Work out the finished part from the listing and answer in its coordinate system (mm). A direction names the side the tool comes from. Coordinates: 2 decimals unless noted, no trailing zeros. Order: outer loops, then holes, each group sorted by start corner. A loop starts at its lowest first (then second) coordinate and runs counter-clockwise, first axis right, second up.
1. The part is cut by section C-C, the plane z = -23.5. Give the vertices of the cut face in (x, y), then the cut area to 3 significant figures.
2. Find the intervals of material crossed by probe 1 along Y at (x, z) = (-29, -1.5); probe 2 along Z at (x, y) = (4.5, -23); probe 3 along Z at (x, y) = (6.5, -37.5), in increasing order.
3. Flat-ended cylindrical pins translate along their axes: pin 1 Ø2.5 at (y, z) = (-8, 23.5) entering from +X; pin 2 Ø3 at (x, z) = (15.34, 2.19) entering from +Y; pin 3 Ø2 at (x, y) = (-28.5, -6) entering from -Z; pin 4 Ø1.5 at (x, y) = (-9.5, -8) entering from +Z. Find the tip coordinate at first contact, or state that the pin passes through.
4. A tool of negligible diameter and unlimited length cuts with its end or side. For faces 1 (the flat face through (3.5, -38, 24)), 2 (the flat face through (16.084, 2, 14)), 3 (the flat face through (-32.5, -6, 0)), from which of +Z, -Z, +X, -X, +Y, -Y can it reach the whole face along a straight path? Write none if from no direction.
5. The part is cut by section D-D, the plane y = -4. Give the vertices of the cut face in (x, z).
6. The part is cut by section B-B, the plane y = -38. Give the vertices of the cut face in (x, z).
7. The part is cut by section A-A, the plane x = -5.5. Give the vertices of the cut face in (y, z), then the cut area to 3 significant figures.
8. Determine the mould class of faces 4 (the flat face through (-29, -20, 0)), 5 (the flat face through (-30, -6, -10)), 6 (the flat face through (9, -23, -18.5)) for opening direction Z: +Z half, -Z half, draft (parallel to the pull), parting line (faces both ways), or undercut.
Autodesk Inventor part; units mm, degrees
ref_plane "YZ Plane" through (0, 0, 0) normal (1, 0, 0) x (0, 1, 0)
ref_plane "XZ Plane" through (0, 0, 0) normal (0, 1, 0) x (-1, 0, 0)
ref_plane "XY Plane" through (0, 0, 0) normal (0, 0, 1) x (1, 0, 0)
sketch "Sketch1" plane through (0, 0, 0) normal (0, 1, 0) x (-1, 0, 0)
  circle A0 centre (0, 0) radius 18.5
  line L0 (5.5131, -10.5135) -> (5.5131, 1.8865)
  circle A1 centre (5.5131, -4.3135) radius 6.2
  line L1 (0, 0) -> (-24.4, 0)
  circle A2 centre (5.5131, -4.3135) radius 3
  circle A3 centre (5.5131, -4.3135) radius 40
  line L2 (-24.4, 0) -> (-24.4, -81.1676)
  line L3 (-24.4, -81.1676) -> (-24.4, 62.3764)
  line L4 (0, 0) -> (0, 28.5)
  line L5 (18.5, 0) -> (28.5, 0)
  line L6 (0, -18.5) -> (0, -28.5)
  arc A4 (28.5, 0) -> (0, 28.5) centre (0, 0) ccw
  arc A5 (0, -28.5) -> (28.5, 0) centre (0, 0) ccw
  line L7 (0, 18.5) -> (0, 23.5)
  line L8 (0, 18.5) -> (-18.5, 18.5)
  line L9 (-18.5, 18.5) -> (-18.5, 28.5)
  line L10 (-18.5, 28.5) -> (0, 28.5)
  line L11 (0, -18.5) -> (-18.5, -18.5)
  line L12 (-18.5, -18.5) -> (-18.5, -28.5)
  line L13 (-18.5, -28.5) -> (0, -28.5)
  line L14 (5.5131, -4.3135) -> (-72.1542, -4.3135)
  line L15 (0, 0) -> (5.5051, -4.3135)
  line L16 (0, 0) -> (6.9938, 0) construction
  line L17 (-16.0843, 18.5) -> (-16.0843, -18.5)
  circle A6 centre (0, 0) radius 15.5
  circle A7 centre (5.5051, -4.3135) radius 24.193
  circle A8 centre (5.5051, -4.3135) radius 10.066
  circle A9 centre (15.3445, -2.1897) radius 1.75
  circle A10 centre (9.5686, 12.1939) radius 1.75
  circle A11 centre (-5.7759, 14.3836) radius 1.75
  circle A12 centre (-15.3445, 2.1897) radius 1.75
  circle A13 centre (-9.5686, -12.1939) radius 1.75
  circle A14 centre (5.7759, -14.3836) radius 1.75
  point P0 (-17.3596, -28.5)
  point P1 (-18.5, -27.6751)
  point P2 (-17.3622, 28.5)
  point P3 (-18.5, 27.6767)
  point P4 (-16.0843, -9.1402)
  point P5 (-16.0843, 9.1402)
  dimension "d59" = 31
  dimension "d65" = 20.132
  dimension "d2" = 12.4
  dimension "d4" = 6
  dimension "d5" = 80
  dimension "d13" = 7
  dimension "d14" = 24.4
  dimension "d17" = 37
  dimension "d18" = 28.5
  dimension "d19" = 10
  dimension "d20" = 10
  dimension "d58" = 38.08
  dimension "d63" = 48.386
  dimension "d66" = 3.5
  dimension "d69" = 360
extrude "Extrusion1" add sketch "Sketch1" along normal blind 4 contours A0 L17 L14 A6 A13 A14 A8 A9 A10 L4 | L5 A5 A7 L6 A0 | A0 L4 A7 A4 L5 | L4 A6 A11 A12 L17 A7 A0 | L8 A7 L4 | A0 A7 L8 | L11 A7 L17 A0 | L6 A7 L11 | A7 L17 A0 | A0 L17 L8 A7 | A6 A10 A9 A8 L4 | L4 A8 L1 A6 A12 A11 | A7 L8 L9 A3 L10 L4 | L4 A4 A7 | A0 L14 L17 | A7 A5 L6 | L6 L13 L12 L11 A7 | L11 L17 A7 | L17 A7 L1 A0 | L17 A12 L1 A7 | A8 A9 A6 A14 L14 A1 L15 L4 | L4 L1 A8 | A0 A7 L1 L17 L14 | L17 L1 A6 L14 | L1 A7 A0 | L15 A1 L14 A8 L1 | A8 L14 A6 L1 | L14 A8 A14 A6 A13 | L17 A12 A6 L1 | A3 L9 L10 | A9 A8 A14 A6
extrude "Extrusion2" add sketch "Sketch1" against normal blind 50 contours L5 A5 A7 L6 A0 | A0 L4 A7 A4 L5 | L8 A7 L4 | L6 A7 L11 | A7 L8 L9 A3 L10 L4 | L4 A4 A7 | A7 A5 L6 | L6 L13 L12 L11 A7 | A3 L9 L10
sketch "Sketch2" plane through (18.5, 4, 28.5) normal (1, 0, 0) x (0, 0, -1)
  point P0 (28.5, -4)
ref_plane "Work Plane1" through (0, -22, 0) normal (0, 1, 0) x (1, 0, 0)
sketch "Sketch5" plane through (0, -22, 0) normal (0, 1, 0) x (1, 0, 0)
  arc A0 (0, 28.5) -> (0, -28.5) centre (0, 0) ccw
  line L0 (-28.5, 0) -> (-28.5, -10)
  line L1 (-28.5, -10) -> (-28.5, 10)
  line L2 (-28.5, 10) -> (-23.5, 10)
  line L3 (-23.5, 10) -> (-23.5, -10)
  line L4 (-23.5, -10) -> (-28.5, -10)
  line L5 (-28.5, -10) -> (-33.5, -10)
  line L6 (-33.5, -10) -> (-33.5, 10)
  line L7 (-33.5, 10) -> (-28.5, 10)
  line L8 (-28.5, 10) -> (-28.5, 7)
  line L9 (-28.5, 7) -> (-29.5, 7)
  line L10 (-29.5, 7) -> (-32.5, 7)
  line L11 (-32.5, 7) -> (-33.5, 7)
  line L12 (-28.5, -10) -> (-28.5, -7)
  line L13 (-28.5, -7) -> (-29.5, -7)
  line L14 (-29.5, -7) -> (-32.5, -7)
  line L15 (-32.5, -7) -> (-33.5, -7)
  line L16 (-33.5, -7) -> (-33.5, 7)
  line L17 (-32.5, -7) -> (-32.5, 7)
  line L18 (-29.5, -7) -> (-29.5, 7)
  point P0 (0, 0)
  point P1 (-26.688, 10)
  point P2 (-26.688, -10)
  dimension "d31" = 10
  dimension "d32" = 20
  dimension "d33" = 5
  dimension "d34" = 5
  dimension "d35" = 3
  dimension "d36" = 1
  dimension "d37" = 3
  dimension "d38" = 3
  dimension "d39" = 1
  dimension "d40" = 3
  dimension "d41" = 1
extrude "Extrusion3" add sketch "Sketch5" along normal blind 2 contours A0 L1 L2 | A0 L4 L0 | L0 L13 L18 L9 L1 | L1 L9 L10 L11 L6 L7 | L0 L5 L6 L15 L14 L13 | L11 L17 L15 L6
pattern_linear "Rectangular Pattern1" count 2 spacing 15 along (0, 1, 0) of "Extrusion3"
pattern_linear "Rectangular Pattern2" count 2 spacing 15 along (0, -1, 0) of "Extrusion3"
sketch "Sketch6" plane through (18.5, 4, 28.5) normal (1, 0, 0) x (0, 0, -1)
  line L0 (57, 0) -> (0, 0)
  line L1 (0, 0) -> (10, 0)
  line L2 (10, 0) -> (5, 0)
  line L3 (5, 0) -> (5, -54)
  line L4 (0, -54) -> (57, -54)
  line L5 (5, -27) -> (5, -12)
  line L6 (5, -12) -> (5, -42)
  circle A0 centre (5, -42) radius 2
  circle A1 centre (5, -12) radius 2
  point P0 (28.5, -4)
  dimension "d50" = 5
  dimension "d51" = 15
  dimension "d52" = 30
  dimension "d53" = 4
  dimension "d54" = 4
extrude "Extrusion4" cut sketch "Sketch6" against normal blind 15
mirror "Mirror1" about plane through (0, 0, 0) normal (0, 0, 1) of "Extrusion4"
sketch "Sketch7" plane through (18.5, 4, 28.5) normal (1, 0, 0) x (0, 0, -1)
  point P0 (28.5, -4)
properties part number "Motor_mount_Right"
Geometry says:
1. outline: (-16.12, -50) - (18.5, -50) - (18.5, -40) - (3.5, -40) - (3.5, -36) - (18.5, -36) - (18.5, -10) - (3.5, -10) - (3.5, -6) - (18.5, -6) - (18.5, 4) - (-16.12, 4) - close
1. area: 1,750 mm2
2. probe 1: y = -37 to -35, -22 to -20, -7 to -5
2. probe 2: z = -28.5 to -18.5, 18.5 to 28.5
2. probe 3: z = -28.5 to -25.44, -21.56 to -18.5, 18.5 to 21.56, 25.44 to 28.5
3. pin 1: stops at x = 3.5
3. pin 2: passes through
3. pin 3: stops at z = -10
3. pin 4: stops at z = 27.12
4. face 1: +X
4. face 2: +X, +Y, -Y
4. face 3: +Y, -Y
5. outline: (0, -28.5) - (18.5, -28.5) - (18.5, -18.5) - (0, -18.5) arc R18.5 cw to (0, 18.5) - (18.5, 18.5) - (18.5, 28.5) - (0, 28.5) arc R28.5 ccw to start
6. outline: (0, -28.5) - (18.5, -28.5) - (18.5, -25.5) - (3.5, -25.5) - (3.5, -21.5) - (18.5, -21.5) - (18.5, -18.5) - (0, -18.5) arc R18.5 cw to (0, 18.5) - (18.5, 18.5) - (18.5, 21.5) - (3.5, 21.5) - (3.5, 25.5) - (18.5, 25.5) - (18.5, 28.5) - (0, 28.5) arc R28.5 ccw to start
7. outline: (-50, -27.96) - (4, -27.96) - (4, -16.11) - (0, -16.11) - (0, -17.66) - (-50, -17.66) - close; (-50, 17.66) - (0, 17.66) - (0, 1.89) - (4, 1.89) - (4, 27.96) - (-50, 27.96) - close; (0, -12.66) - (4, -12.66) - (4, -10.51) - (0, -10.51) - close
7. area: 1,190 mm2
8. face 4: draft
8. face 5: -Z half
8. face 6: undercut
